For this review, use the dimensioned drawing (mm, ordinates from the lowest corner) and the shaded views. A direction names the side the tool comes from. Coordinates: 2 decimals unless noted, no trailing zeros. Loops run counter-clockwise (first coordinate to the right, second up) from the corner with the lowest first, then second, coordinate; pieces in that order, holes last. Notation, with made-up numbers: (6.5, 64.5) - (23.5, 64.5) arc R30 cw to (23.5, 94.5) - close; hole circle Ø8 at (65.5, -6.5). An arc over 180 degrees is marked (long way). Answer in a Markdown table with one row per item. Add a question column.
(1) We need section A-A on x = 3.4. Give the number of separate pieces and of enclosed holes in the cut face.
(2) We need section D-D on z = 13.75. Write out the cut boundary in (x, y) (1 decimal).
(3) Machinability: for the marked faces 1, 2 and 3, which of the approach directions +Z, -Z, +X, -X, +Y, -Y give a long, thin tool a straight path to every point of the face, cutting with its end or side? Answer none if there is none.
(4) We need section B-B on z = 5.75. Write out the cut boundary in (x, y) (1 decimal).
(5) For line 1 along Z through (x, y) = (0.6, 6); line 2 along Z through (x, y) = (1.2, 7.25); line 3 along X through (y, z) = (8, 3.25) (1 decimal), list the stretches that pass through material, from the lowest coordinate up.
(6) For P1, Ø5, axis at y = 8, z = 10.5, coming from the +X side; P2, Ø1.5, axis at x = 2, y = 8, coming from the +Z side; P3, Ø1.1, axis at x = 2, y = 5, coming from the -Z side; P4, Ø2, axis at y = 4.5, z = 6.5, coming from the -X side, all flat-tipped, find the tip position at first contact; note any pin that passes through.
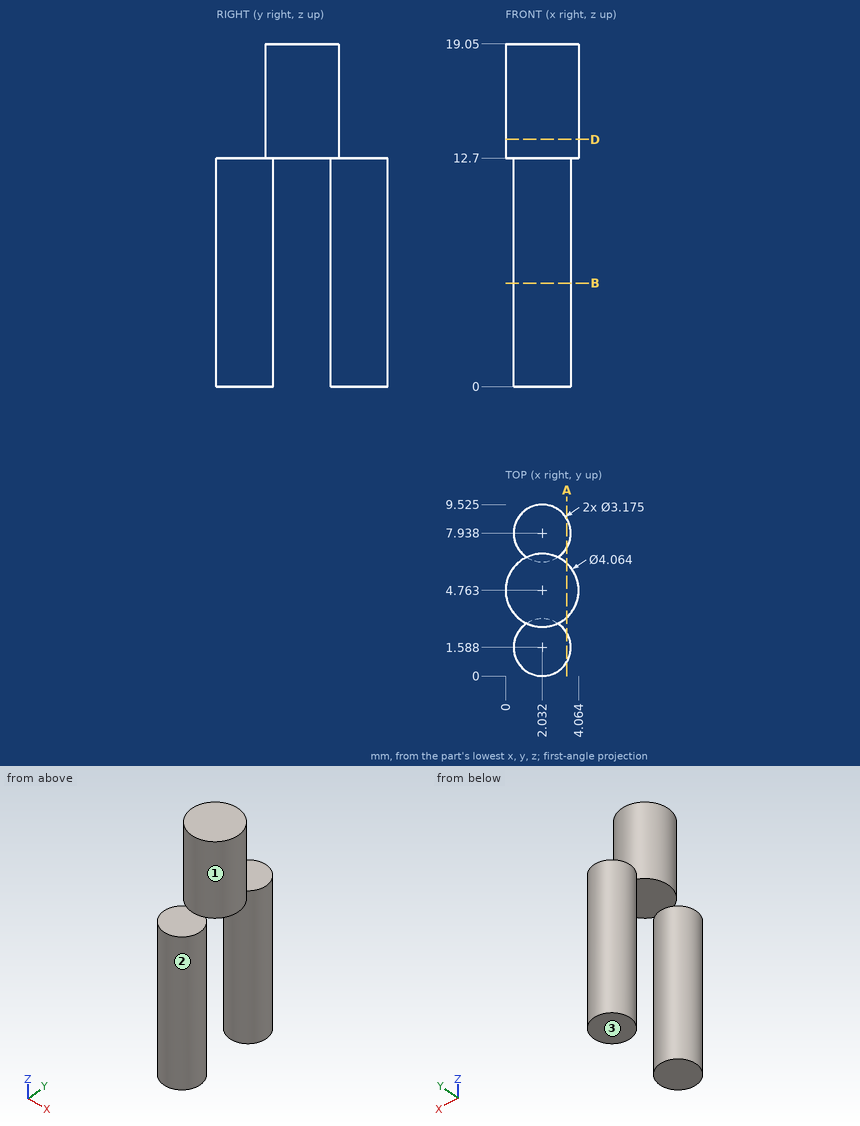
Outcome:
| question | item | result |
|---|---|---|
| 1 | separate pieces | 3 |
| 1 | enclosed holes | 0 |
| 2 | outline | circle Ø4.1 at (2, 4.8) |
| 3 | face 1 | +Z |
| 3 | face 2 | -Z |
| 3 | face 3 | -Z, +X, -X, +Y, -Y |
| 4 | outline | circle Ø3.2 at (2, 1.6); circle Ø3.2 at (2, 7.9) |
| 5 | line 1 | 12.7 to 19.05 |
| 5 | line 2 | 0 to 12.7 |
| 5 | line 3 | 0.4 to 3.6 |
| 6 | P1 | x = 3.62 |
| 6 | P2 | z = 12.7 |
| 6 | P3 | z = 12.7 |
| 6 | P4 | through |
